Can you work these out from the model? Positions are in its coordinate system, mm. Face numbers are marked on the shaded views. A direction names the side the tool comes from. Coordinates: 2 decimals unless noted, no trailing zeros. Order: outer loops, then holes, each group sorted by start corner. A loop starts at its lowest first (then second) coordinate and runs counter-clockwise, first axis right, second up. Notation, with made-up numbers: (42, 82) -> (65, 82) arc R15 ccw to (65, 89) -> close; hole circle Ø8 at (33, -18). An arc over 180 degrees is marked (long way). Answer as CSV lines item,"result".
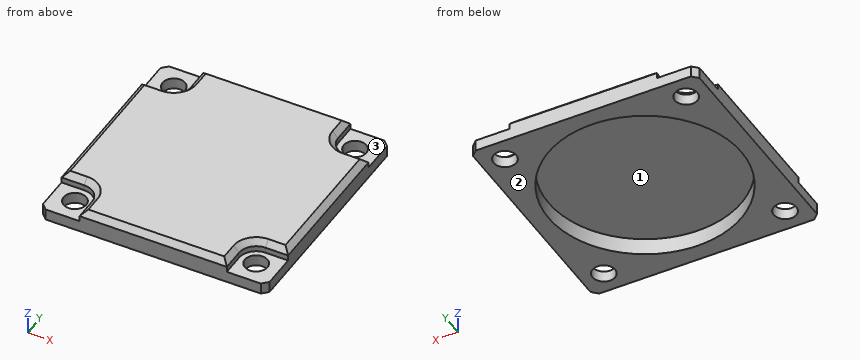
from build123d import *

# Parameters (mm, degrees)
CROQUIS1_W              = 40
CROQUIS1_H              = 40
CROQUIS1_R              = 2
CROQUIS1_R_2            = 17
SALIENTE_EXTRUIR1_DEPTH = 3
CROQUIS2_W              = 40
CROQUIS2_H              = 40
SALIENTE_EXTRUIR2_DEPTH = 1
CORTAR_EXTRUIR1_DEPTH   = 2
CHAFL_N1_SIZE           = 1


with BuildPart() as part:
    # Croquis1 → Saliente-Extruir1 (new body)
    with BuildSketch(Plane.XY):
        Rectangle(CROQUIS1_W, CROQUIS1_H)
        with Locations((-16, -16)):
            Circle(CROQUIS1_R, mode=Mode.SUBTRACT)
        with Locations((16, -16)):
            Circle(CROQUIS1_R, mode=Mode.SUBTRACT)
        with Locations((16, 16)):
            Circle(CROQUIS1_R, mode=Mode.SUBTRACT)
        with Locations((-16, 16)):
            Circle(CROQUIS1_R, mode=Mode.SUBTRACT)
        Circle(CROQUIS1_R_2, mode=Mode.SUBTRACT)
    extrude(amount=SALIENTE_EXTRUIR1_DEPTH)

    # Croquis2 → Saliente-Extruir2 (add)
    with BuildSketch(Plane.XY.offset(3)):
        Rectangle(CROQUIS2_W, CROQUIS2_H)
    extrude(amount=SALIENTE_EXTRUIR2_DEPTH)

    # Croquis3 → Cortar-Extruir1 (cut)
    with BuildSketch(Plane.XY.offset(4)):
        with BuildLine():
            Line((13, 16), (13, 20))
            Line((13, 20), (20, 20))
            Line((20, 20), (20, 13))
            Line((20, 13), (16, 13))
            ThreePointArc((16, 13), (13.878679656, 13.878679656), (13, 16))
        make_face()
        with BuildLine():
            Line((-13, 16), (-13, 20))
            Line((-13, 20), (-20, 20))
            Line((-20, 20), (-20, 13))
            Line((-20, 13), (-16, 13))
            ThreePointArc((-16, 13), (-13.878679656, 13.878679656), (-13, 16))
        make_face()
        with BuildLine():
            Line((16, -13), (20, -13))
            Line((20, -13), (20, -20))
            Line((20, -20), (13, -20))
            Line((13, -20), (13, -16))
            ThreePointArc((13, -16), (13.878679656, -13.878679656), (16, -13))
        make_face()
        with BuildLine():
            Line((-13, -16), (-13, -20))
            Line((-13, -20), (-20, -20))
            Line((-20, -20), (-20, -13))
            Line((-20, -13), (-16, -13))
            ThreePointArc((-16, -13), (-13.878679656, -13.878679656), (-13, -16))
        make_face()
    extrude(amount=-CORTAR_EXTRUIR1_DEPTH, mode=Mode.SUBTRACT)

    # Chaflán1
    chafl_n1_edges = [part.edges().sort_by_distance(p)[0] for p in [
        (-20, 0, 4),
        (0, -20, 4),
        (20, 0, 4),
        (0, 20, 4),
        (20, -20, 1),
        (-20, -20, 1),
        (-20, 20, 1),
        (20, 20, 1),
        (-13.878679656, -13.878679656, 4),
        (-18, -13, 4),
        (-13, -18, 4),
        (13.878679656, -13.878679656, 4),
        (13, -18, 4),
        (18, -13, 4),
        (13.878679656, 13.878679656, 4),
        (18, 13, 4),
        (13, 18, 4),
        (-18, 13, 4),
        (-13.878679656, 13.878679656, 4),
        (-13, 18, 4),
    ]]
    chamfer(chafl_n1_edges, length=CHAFL_N1_SIZE)


solid = part.part
Q1. If I drill on line 1 (Z direction, x = 4, y = 14.5); line 2 (X direction, y = -17.5, z = 0.75); line 3 (Y direction, x = -0.5, z = 2.4), over which ranges is the centre line in solid material (lowest first)?
Solution:
line 1,"3 to 4"
line 2,"-20 to -17.32, -14.68 to 14.68, 17.32 to 20"
line 3,"-20 to -16.99, 16.99 to 20"
Q2. Imagine slicing it at B-B (y = 16.5). List the corners of the cut face in (x, z) for me, and give its area (3 significant figures).
Solution:
outline,"(-20, 0) -> (-17.94, 0) -> (-17.94, 2) -> (-20, 2) -> close; (-14.06, 0) -> (-4.09, 0) -> (-4.09, 3) -> (4.09, 3) -> (4.09, 0) -> (14.06, 0) -> (14.06, 2) -> (13, 2) -> (13, 3) -> (12, 4) -> (-12, 4) -> (-13, 3) -> (-13, 2) -> (-14.06, 2) -> close; (17.94, 0) -> (20, 0) -> (20, 2) -> (17.94, 2) -> close"
area,"91.0 mm2"
Q3. Which directions (+Z, -Z, +X, -X, +Y, -Y) give clear straight access to the entire face, cutting with the end or side of a thin tool? Please do the marked faces 1, 2 and 3.
Solution:
face 1,"-Z"
face 2,"-Z, +X, -X, +Y, -Y"
face 3,"+Z, +X, +Y"
Q4. For P1, Ø20.5, axis at x = 0, y = 0, coming from the -Z side; P2, Ø3, axis at x = -16, y = -16, coming from the +Z side; P3, Ø0.8, axis at x = -17.5, z = 2.5, coming from the -Y side; P4, Ø6.5, axis at x = 16, y = -16, coming from the +Z side, each with a flat end and sliding along its axis, tell me the tip position at first contact or that it passes through.
Solution:
P1,"z = 3"
P2,"through"
P3,"y = -13"
P4,"z = 3.25"
Q5. Imagine slicing it at A-A (z = 0.5). List the corners of the cut face in (x, y) for me, and give its area (3 significant figures).
Solution:
outline,"(-20, -19) -> (-19, -20) -> (19, -20) -> (20, -19) -> (20, 19) -> (19, 20) -> (-19, 20) -> (-20, 19) -> close; hole circle Ø4 at (-16, -16); hole circle Ø4 at (-16, 16); hole circle Ø34 at (0, 0); hole circle Ø4 at (16, -16); hole circle Ø4 at (16, 16)"
area,"640 mm2"
Q6. Imagine slicing it at C-C (y = 0). List the corners of the cut face in (x, z) for me.
Solution:
outline,"(-20, 0) -> (-17, 0) -> (-17, 3) -> (17, 3) -> (17, 0) -> (20, 0) -> (20, 3) -> (19, 4) -> (-19, 4) -> (-20, 3) -> close"
